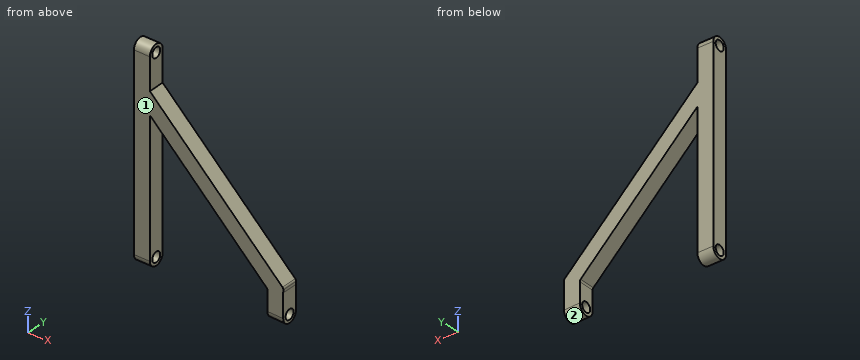
from build123d import *

# Parameters (mm, degrees)
CROQUIS1_R                 = 12.5
SALIENTE_EXTRUIR1_DEPTH    = 40
SALIENTE_EXTRUIR2_DEPTH    = 40
CORTAR_EXTRUIR2_DEPTH      = 45
CORTAR_EXTRUIR2_DEPTH_BACK = 45
CROQUIS3_R                 = 12.5


with BuildPart() as part:
    # Croquis1 → Saliente-Extruir1 (new body)
    with BuildSketch(Plane(origin=(0, 0, 0), x_dir=(0, 0, -1), z_dir=(1, 0, 0))):
        with BuildLine():
            ThreePointArc((0, 20), (-20, 0), (0, -20))
            Line((0, -20), (475, -20))
            ThreePointArc((475, -20), (495, 0), (475, 20))
            Line((475, 20), (0, 20))
        make_face()
        Circle(CROQUIS1_R, mode=Mode.SUBTRACT)
        with Locations(Location((475, 0, 0), (0, 0, 180))):
            Circle(CROQUIS1_R, mode=Mode.SUBTRACT)
    extrude(amount=SALIENTE_EXTRUIR1_DEPTH)

    # Croquis2 → Saliente-Extruir2 (add)
    with BuildSketch(Plane(origin=(0, 20, 0), x_dir=(1, 0, 0), z_dir=(0, 1, 0))):
        with BuildLine():
            Line((40, 135.706571889), (40, 80))
            Line((40, 80), (372.872939005, 402.648821131))
            ThreePointArc((372.872939005, 402.648821131), (374.476832278, 405.021700465), (374.992889328, 407.83891808))
            Line((374.992889328, 407.83891808), (374.806076613, 415.181628683))
            Line((374.806076613, 415.181628683), (374.806076613, 495))
            Line((374.806076613, 495), (335.193923387, 495))
            Line((335.193923387, 495), (335.193923387, 462.022456719))
            Line((335.193923387, 462.022456719), (335.193923387, 424.789203994))
            ThreePointArc((335.193923387, 424.789203994), (334.64151447, 422.067558315), (333.071714854, 419.776654567))
            Line((333.071714854, 419.776654567), (40, 135.706571889))
        make_face()
    extrude(amount=-SALIENTE_EXTRUIR2_DEPTH)

    # Croquis3 → Cortar-Extruir2 (cut, two sides: drawn at the far end of the back side and taken through both)
    with BuildSketch(Plane(origin=(385.119812841, 0, -9.798190532), x_dir=(-0.025433697775531394, 0, -0.9996765111862251), z_dir=(0.9996765111862251, 0, -0.025433697775531394)).offset(-CORTAR_EXTRUIR2_DEPTH_BACK)):
        with Locations(Location((465.30716856, 0, 0), (0, 0, 180))):
            Circle(CROQUIS3_R)
        with BuildLine():
            Line((465.30716856, 20), (485.30716856, 20))
            Line((485.30716856, 20), (531.151017537, 20))
            Line((531.151017537, 20), (531.151017537, -20))
            Line((531.151017537, -20), (485.30716856, -20))
            Line((485.30716856, -20), (465.30716856, -20))
            ThreePointArc((465.30716856, -20), (485.30716856, 0), (465.30716856, 20))
        make_face()
    extrude(amount=CORTAR_EXTRUIR2_DEPTH + CORTAR_EXTRUIR2_DEPTH_BACK, mode=Mode.SUBTRACT)


solid = part.part
Could you check a few things on this model? Use its own coordinates, in mm. Face numbers are marked on the shaded views. Round coordinates to 2 decimals unless told otherwise and drop trailing zeros. Loops run counter-clockwise (first coordinate to the right, second up) from the corner with the lowest first, then second, coordinate; pieces in that order, holes last. Notation, with made-up numbers: (-36.75, 26.5) - (-1.75, 26.5) arc R18 ccw to (-1.75, 32.5) - close; hole circle Ø11 at (-39, 40). An arc over 180 degrees is marked (long way). Write item = value, one per line.
1) If we mould it in two halves opening along X, with no side actions, what happens to the marked faces 1 and 2? For each: pulls with the +X half, pulls with the -X half, needs draft (parallel to the pull), parting line crosses it, or undercut.
Computed:
face_1 = needs draft
face_2 = undercut
2) Imagine slicing it at D-D (x = 275.5). Please give me the cut outline in (y, z).
Computed:
outline = (-20, -363.97) - (20, -363.97) - (20, -308.27) - (-20, -308.27) - close
3) I need wall thicknesses on line 1 along X through (y, z) = (9.5, -435.5); line 2 along X through (y, z) = (16.5, -382); line 3 along X through (y, z) = (-4.5, -44). Which ranges of each line are inside material? Lowest first, please. Write a range as from..to.
Computed:
line_1 = 0..40, 335.19..374.81
line_2 = 0..40, 294.1..351.57
line_3 = 0..40
4) Imagine slicing it at A-A (z = -434). Please give me the cut outline in (x, y).
Computed:
outline = (0, -20) - (40, -20) - (40, 20) - (0, 20) - close; (335.19, -20) - (374.81, -20) - (374.81, 20) - (335.19, 20) - close
5) Imagine slicing it at C-C (z = -54). Please give me the cut outline in (x, y).
Computed:
outline = (0, -20) - (40, -20) - (40, 20) - (0, 20) - close
6) I'm going to push flat-ended pins straight in: P1, Ø1, axis at x = 192.5, y = -15.5, coming from the -Z side; P2, Ø6, axis at y = 11.5, z = -376, coming from the +X side; P3, Ø10, axis at y = 10.5, z = -259.5, coming from the +X side. Where does each tip first touch, or does it pass through?
Computed:
P1 = -284.01
P2 = 348.47
P3 = 230.35
7) Imagine slicing it at B-B (y = 6). Please give me the cut outline in (x, z), and give its area (3 significant figures).
Computed:
outline = (0, -494.08) - (40, -494.08) - (40, -485.97) - (0, -485.97) - close; (0, -464.03) - (40, -464.03) - (40, -135.71) - (333.07, -419.78) arc R6.98 cw to (335.19, -424.79) - (335.19, -463.02) - (374.81, -464.02) - (374.81, -415.18) - (374.99, -407.84) arc R6.98 ccw to (372.87, -402.65) - (40, -80) - (40, -10.97) - (0, -10.97) - close; (0, 10.97) - (40, 10.97) - (40, 19.08) - (0, 19.08) - close; (335.19, -493.07) - (374.81, -494.08) - (374.81, -485.96) - (335.19, -484.96) - close
area = 38,600 mm2
